from build123d import *

# Parameters (mm, degrees)
BASE_FLANGE1_DEPTH = 1
SKETCH6_R          = 27.45
CUT_EXTRUDE1_DEPTH = 10
SKETCH8_R          = 2.05
SKETCH8_R_2        = 1.25
CUT_EXTRUDE2_DEPTH = 10
CIRPATTERN1_COUNT  = 4


# Sheet-metal steps are written as plain solids
with BuildPart() as part:
    # Sketch1 → Base-Flange1 (new body)
    with BuildSketch(Plane(origin=(0, 0, 0), x_dir=(1, 0, 0), z_dir=(0, 1, 0))):
        with BuildLine():
            Line((-46.2, -51.2), (46.2, -51.2))
            ThreePointArc((46.2, -51.2), (49.735533906, -49.735533906), (51.2, -46.2))
            Line((51.2, -46.2), (51.2, 46.2))
            ThreePointArc((51.2, 46.2), (49.735533906, 49.735533906), (46.2, 51.2))
            Line((46.2, 51.2), (-46.2, 51.2))
            ThreePointArc((-46.2, 51.2), (-49.735533906, 49.735533906), (-51.2, 46.2))
            Line((-51.2, 46.2), (-51.2, -46.2))
            ThreePointArc((-51.2, -46.2), (-49.735533906, -49.735533906), (-46.2, -51.2))
        make_face()
    extrude(amount=-BASE_FLANGE1_DEPTH)

    # Sketch6 → Cut-Extrude1 (cut)
    with BuildSketch(Plane(origin=(0, 0, 0), x_dir=(1, 0, 0), z_dir=(0, 1, 0))):
        with Locations(Location((0, 0, 0), (0, 0, 270))):
            Circle(SKETCH6_R)
    extrude(amount=-CUT_EXTRUDE1_DEPTH, mode=Mode.SUBTRACT)

    # Sketch8 → Cut-Extrude2 (cut)
    with BuildSketch(Plane(origin=(0, 0, 0), x_dir=(1, 0, 0), z_dir=(0, 1, 0))):
        with Locations(Location((40.45, 40.45, 0), (0, 0, 270))):
            Circle(SKETCH8_R)
        with Locations(Location((34.95, 34.95, 0), (0, 0, 270))):
            Circle(SKETCH8_R_2)
    cut_extrude2 = extrude(amount=-CUT_EXTRUDE2_DEPTH, mode=Mode.SUBTRACT)

    # CirPattern1: Cut-Extrude2 ×4 about axis
    cirpattern1_axis = Axis((0, 0, 0), (0, 1, 0))
    for i in range(1, CIRPATTERN1_COUNT):
        add(cut_extrude2.rotate(cirpattern1_axis, i * 360 / CIRPATTERN1_COUNT), mode=Mode.SUBTRACT)


solid = part.part
Verification items for the finished model (mm, model axes). Give positions to 0.01 mm unless a question says otherwise; leave off trailing zeros. Order: outer loops, then holes, each group sorted by start corner. A loop starts at its lowest first (then second) coordinate and runs counter-clockwise, first axis right, second up. Notation, with made-up numbers: M 61.5,85.5 L 70.5,85.5 A14 cw 70.5,97.5 Z; hole C 29,-9.75 d3. An arc over 180 degrees is marked long. Use one line per item in the form item = value. Start each with the question number.
Q1. Scan lines: line 1 along X through (y, z) = (-0.2, -40.45); line 2 along X through (y, z) = (-0.25, -34.95); line 3 along X through (y, z) = (-0.2, 0). Record each from-to range of solid material in increasing order. Write a range as [from, to].
Q2. Section check A-A (z = 0). Enter the section's corners in (x, y), then the cut area to 3 significant figures.
Q3. Section check B-B (x = 0). Enter the section's corners in (y, z), then the cut area to 3 significant figures.
Q4. Section check D-D (y = -0.7). Count the separate pieces of the cut face and the enclosed holes in it, then the cut area to 3 significant figures.
Q5. Go/stop test with a flat-tipped pin: pin 1 Ø3.5 at (x, z) = (40.45, 40.45) entering from -Y. Record where the tip stops, or that it passes through.
Q6. Mould release check, pull along Z, two halves, no side actions. Record for faces 1 (the flat face through (22, 0, 22)), 2 (the cylindrical face through (49.7, -0.49, 49.77)), 3 (the cylindrical face through (8.25, -0.49, 26.18)): +Z half, -Z half, draft (parallel to the pull), parting line (faces both ways), or undercut.
Q7. Section check C-C (z = 40.45). Enter the section's corners in (x, y), then the cut area to 3 significant figures.
Evaluation:
q1.line_1 = [-51.2, -42.5], [-38.4, 38.4], [42.5, 51.2]
q1.line_2 = [-51.2, -36.2], [-33.7, 33.7], [36.2, 51.2]
q1.line_3 = [-51.2, -27.45], [27.45, 51.2]
q2.outline = M -51.2,-1 L -27.45,-1 L -27.45,0 L -51.2,0 Z; M 27.45,-1 L 51.2,-1 L 51.2,0 L 27.45,0 Z
q2.area = 47.5 mm2
q3.outline = M -1,-51.2 L 0,-51.2 L 0,-27.45 L -1,-27.45 Z; M -1,27.45 L 0,27.45 L 0,51.2 L -1,51.2 Z
q3.area = 47.5 mm2
q4.separate_pieces = 1
q4.enclosed_holes = 9
q4.area = 8,020 mm2
q5.pin_1 = through
q6.face_1 = draft
q6.face_2 = +Z half
q6.face_3 = undercut
q7.outline = M -51.2,-1 L -42.5,-1 L -42.5,0 L -51.2,0 Z; M -38.4,-1 L 38.4,-1 L 38.4,0 L -38.4,0 Z; M 42.5,-1 L 51.2,-1 L 51.2,0 L 42.5,0 Z
q7.area = 94.2 mm2
